from build123d import *

# Parameters (mm, degrees)
F1_DEPTH = 54


with BuildPart() as f1:
    # F0 (on Top) → F1 (new body)
    with BuildSketch(Plane.XY):
        with BuildLine():
            ThreePointArc((-4, 12.4743737318), (0, 13.1), (4, 12.4743737318))
            Line((4, 12.4743737318), (4, 25.1843205189))
            Line((4, 25.1843205189), (-4, 25.1843205189))
            Line((-4, 25.1843205189), (-4, 12.4743737318))
        make_face()
        with BuildLine():
            Line((-4, 25.1843205189), (4, 25.1843205189))
            ThreePointArc((4, 25.1843205189), (0, 25.5), (-4, 25.1843205189))
        make_face()
        with BuildLine():
            ThreePointArc((25.5, 0), (25.4209576259, 2.0062186779), (25.1843205189, 4))
            Line((25.1843205189, 4), (25.1843205189, -4))
            ThreePointArc((25.1843205189, -4), (25.4209576259, -2.0062186779), (25.5, 0))
        make_face()
        with BuildLine():
            Line((25.1843205189, 4), (12.4743737318, 4))
            ThreePointArc((12.4743737318, 4), (12.942648413, 2.0243152069), (13.1, 0))
            ThreePointArc((13.1, 0), (12.942648413, -2.0243152069), (12.4743737318, -4))
            Line((12.4743737318, -4), (25.1843205189, -4))
            Line((25.1843205189, -4), (25.1843205189, 4))
        make_face()
        with BuildLine():
            ThreePointArc((-4, -25.1843205189), (0, -25.5), (4, -25.1843205189))
            Line((4, -25.1843205189), (-4, -25.1843205189))
        make_face()
        with BuildLine():
            Line((-25.1843205189, -4), (-25.1843205189, 4))
            ThreePointArc((-25.1843205189, 4), (-25.5, 0), (-25.1843205189, -4))
        make_face()
        with BuildLine():
            ThreePointArc((-12.4743737318, -4), (-13.1, 0), (-12.4743737318, 4))
            Line((-12.4743737318, 4), (-25.1843205189, 4))
            Line((-25.1843205189, 4), (-25.1843205189, -4))
            Line((-25.1843205189, -4), (-12.4743737318, -4))
        make_face()
        with BuildLine():
            Line((4, -25.1843205189), (4, -12.4743737318))
            ThreePointArc((4, -12.4743737318), (0, -13.1), (-4, -12.4743737318))
            Line((-4, -12.4743737318), (-4, -25.1843205189))
            Line((-4, -25.1843205189), (4, -25.1843205189))
        make_face()
        with BuildLine():
            Line((-8.1737384348, 4), (-10.3542261903, 4))
            ThreePointArc((-10.3542261903, 4), (-11.1, 0), (-10.3542261903, -4))
            Line((-10.3542261903, -4), (-8.1737384348, -4))
            ThreePointArc((-8.1737384348, -4), (-9.1, 0), (-8.1737384348, 4))
        make_face()
        with BuildLine():
            ThreePointArc((-10.3542261903, -4), (-11.1, 0), (-10.3542261903, 4))
            Line((-10.3542261903, 4), (-12.4743737318, 4))
            ThreePointArc((-12.4743737318, 4), (-13.1, 0), (-12.4743737318, -4))
            Line((-12.4743737318, -4), (-10.3542261903, -4))
        make_face()
        with BuildLine():
            Line((4, 8.1737384348), (4, 10.3542261903))
            ThreePointArc((4, 10.3542261903), (0, 11.1), (-4, 10.3542261903))
            Line((-4, 10.3542261903), (-4, 8.1737384348))
            ThreePointArc((-4, 8.1737384348), (0, 9.1), (4, 8.1737384348))
        make_face()
        with BuildLine():
            ThreePointArc((-4, 10.3542261903), (0, 11.1), (4, 10.3542261903))
            Line((4, 10.3542261903), (4, 12.4743737318))
            ThreePointArc((4, 12.4743737318), (0, 13.1), (-4, 12.4743737318))
            Line((-4, 12.4743737318), (-4, 10.3542261903))
        make_face()
        with BuildLine():
            ThreePointArc((10.3542261903, 4), (10.9119638634, 2.0344642154), (11.1, 0))
            ThreePointArc((11.1, 0), (10.9119638634, -2.0344642154), (10.3542261903, -4))
            Line((10.3542261903, -4), (12.4743737318, -4))
            ThreePointArc((12.4743737318, -4), (12.942648413, -2.0243152069), (13.1, 0))
            ThreePointArc((13.1, 0), (12.942648413, 2.0243152069), (12.4743737318, 4))
            Line((12.4743737318, 4), (10.3542261903, 4))
        make_face()
        with BuildLine():
            ThreePointArc((10.3542261903, -4), (10.9119638634, -2.0344642154), (11.1, 0))
            ThreePointArc((11.1, 0), (10.9119638634, 2.0344642154), (10.3542261903, 4))
            Line((10.3542261903, 4), (8.1737384348, 4))
            ThreePointArc((8.1737384348, 4), (8.8654108691, 2.052922337), (9.1, 0))
            ThreePointArc((9.1, 0), (8.8654108691, -2.052922337), (8.1737384348, -4))
            Line((8.1737384348, -4), (10.3542261903, -4))
        make_face()
        with BuildLine():
            ThreePointArc((-4, -10.3542261903), (0, -11.1), (4, -10.3542261903))
            Line((4, -10.3542261903), (4, -8.1737384348))
            ThreePointArc((4, -8.1737384348), (0, -9.1), (-4, -8.1737384348))
            Line((-4, -8.1737384348), (-4, -10.3542261903))
        make_face()
        with BuildLine():
            Line((4, -12.4743737318), (4, -10.3542261903))
            ThreePointArc((4, -10.3542261903), (0, -11.1), (-4, -10.3542261903))
            Line((-4, -10.3542261903), (-4, -12.4743737318))
            ThreePointArc((-4, -12.4743737318), (0, -13.1), (4, -12.4743737318))
        make_face()
        with BuildLine():
            Line((-4, 4), (-8.1737384348, 4))
            ThreePointArc((-8.1737384348, 4), (-9.1, 0), (-8.1737384348, -4))
            Line((-8.1737384348, -4), (-4, -4))
            Line((-4, -4), (-4, -2.0615528128))
            ThreePointArc((-4, -2.0615528128), (-4.5, 0), (-4, 2.0615528128))
            Line((-4, 2.0615528128), (-4, 4))
        make_face()
        with BuildLine():
            Line((-4, 4), (-4, 8.1737384348))
            ThreePointArc((-4, 8.1737384348), (-6.4346717088, 6.4346717088), (-8.1737384348, 4))
            Line((-8.1737384348, 4), (-4, 4))
        make_face()
        with BuildLine():
            Line((4, 4), (4, 8.1737384348))
            ThreePointArc((4, 8.1737384348), (0, 9.1), (-4, 8.1737384348))
            Line((-4, 8.1737384348), (-4, 4))
            Line((-4, 4), (-2.0615528128, 4))
            ThreePointArc((-2.0615528128, 4), (0, 4.5), (2.0615528128, 4))
            Line((2.0615528128, 4), (4, 4))
        make_face()
        with BuildLine():
            Line((4, 4), (8.1737384348, 4))
            ThreePointArc((8.1737384348, 4), (6.4346717088, 6.4346717088), (4, 8.1737384348))
            Line((4, 8.1737384348), (4, 4))
        make_face()
        with BuildLine():
            ThreePointArc((9.1, 0), (8.8654108691, 2.052922337), (8.1737384348, 4))
            Line((8.1737384348, 4), (4, 4))
            Line((4, 4), (4, 2.0615528128))
            ThreePointArc((4, 2.0615528128), (4.3732139211, 1.0606601718), (4.5, 0))
            ThreePointArc((4.5, 0), (4.3732139211, -1.0606601718), (4, -2.0615528128))
            Line((4, -2.0615528128), (4, -4))
            Line((4, -4), (8.1737384348, -4))
            ThreePointArc((8.1737384348, -4), (8.8654108691, -2.052922337), (9.1, 0))
        make_face()
        with BuildLine():
            ThreePointArc((-4, -8.1737384348), (0, -9.1), (4, -8.1737384348))
            Line((4, -8.1737384348), (4, -4))
            Line((4, -4), (2.0615528128, -4))
            ThreePointArc((2.0615528128, -4), (0, -4.5), (-2.0615528128, -4))
            Line((-2.0615528128, -4), (-4, -4))
            Line((-4, -4), (-4, -8.1737384348))
        make_face()
        with BuildLine():
            ThreePointArc((-8.1737384348, -4), (-6.4346717088, -6.4346717088), (-4, -8.1737384348))
            Line((-4, -8.1737384348), (-4, -4))
            Line((-4, -4), (-8.1737384348, -4))
        make_face()
        with BuildLine():
            ThreePointArc((4, -8.1737384348), (6.4346717088, -6.4346717088), (8.1737384348, -4))
            Line((8.1737384348, -4), (4, -4))
            Line((4, -4), (4, -8.1737384348))
        make_face()
        with BuildLine():
            Line((2.0615528128, -4), (4, -4))
            Line((4, -4), (4, -2.0615528128))
            ThreePointArc((4, -2.0615528128), (3.1819805153, -3.1819805153), (2.0615528128, -4))
        make_face()
        with BuildLine():
            Line((-4, -2.0615528128), (-4, -4))
            Line((-4, -4), (-2.0615528128, -4))
            ThreePointArc((-2.0615528128, -4), (-3.1819805153, -3.1819805153), (-4, -2.0615528128))
        make_face()
        with BuildLine():
            Line((-2.0615528128, 4), (-4, 4))
            Line((-4, 4), (-4, 2.0615528128))
            ThreePointArc((-4, 2.0615528128), (-3.1819805153, 3.1819805153), (-2.0615528128, 4))
        make_face()
        with BuildLine():
            Line((4, 2.0615528128), (4, 4))
            Line((4, 4), (2.0615528128, 4))
            ThreePointArc((2.0615528128, 4), (3.1819805153, 3.1819805153), (4, 2.0615528128))
        make_face()
    extrude(amount=-F1_DEPTH)


solid = f1.part
Verification items for the finished model (mm, model axes). A direction names the side the tool comes from. Give positions to 0.01 mm unless a question says otherwise; leave off trailing zeros. Order: outer loops, then holes, each group sorted by start corner. A loop starts at its lowest first (then second) coordinate and runs counter-clockwise, first axis right, second up. Notation, with made-up numbers: M 54.25,44.25 L 66.25,44.25 A25 ccw 66.25,63.25 Z; hole C -26,21.5 d10. An arc over 180 degrees is marked long. Use one line per item in the form item = value. Start each with the question number.
Q1. Section check B-B (x = -3). Enter the section's corners in (y, z).
Q2. Section check A-A (z = -41.5). Enter the section's corners in (x, y), then the cut area to 3 significant figures.
Q3. Go/stop test with flat-tipped pins: pin 1 Ø18.5 at (y, z) = (17, -23) entering from -X; pin 2 Ø3 at (x, z) = (11.5, -9.5) entering from -Y; pin 3 Ø13.5 at (y, z) = (-19.5, -25) entering from -X. Record where each tip stops, or that it passes through.
Q4. Scan lines: line 1 along Y through (x, z) = (-11, -45); line 2 along X through (y, z) = (-2, -40). Record each from-to range of solid material in increasing order. Write a range as [from, to].
Q5. Access from +Z, -Z, +X, -X, +Y, -Y to the whole of each face (thin tool, end or side, straight path). Record for faces 1 (the flat face through (17, 4, -27)), 2 (the flat face through (-17, 4, -27)), 3 (the flat face through (-4, -17, -27)), 4 (the flat face through (17, -4, -27)).
Q6. Section check C-C (y = 22.5). Enter the section's corners in (x, z).
Evaluation:
q1.outline = M -25.32,-54 L -3.35,-54 L -3.35,0 L -25.32,0 Z; M 3.35,-54 L 25.32,-54 L 25.32,0 L 3.35,0 Z
q2.outline = M -25.18,-4 L -8.17,-4 A9.1 ccw -4,-8.17 L -4,-25.18 A25.5 ccw 4,-25.18 L 4,-8.17 A9.1 ccw 8.17,-4 L 25.18,-4 A25.5 ccw 25.18,4 L 8.17,4 A9.1 ccw 4,8.17 L 4,25.18 A25.5 ccw -4,25.18 L -4,8.17 A9.1 ccw -8.17,4 L -25.18,4 A25.5 ccw Z; hole C 0,0 d9
q2.area = 728 mm2
q3.pin_1 = -4.77
q3.pin_2 = -4
q3.pin_3 = -4
q4.line_1 = [-4, 4]
q4.line_2 = [-25.42, -4.03], [4.03, 25.42]
q5.face_1 = +Z, -Z, +X, +Y
q5.face_2 = +Z, -Z, -X, +Y
q5.face_3 = +Z, -Z, -X, -Y
q5.face_4 = +Z, -Z, +X, -Y
q6.outline = M -4,-54 L 4,-54 L 4,0 L -4,0 Z
